from build123d import *

# Parameters (mm, degrees)
F0_W      = 36
F0_H      = 54
F1_DEPTH  = 15
F2_W      = 36
F2_H      = 7
F3_DEPTH  = 44
F4_R      = 15
F5_DEPTH  = 22
F7_D      = 20
F8_W      = 5
F8_H      = 7
F9_DEPTH  = 9999
F10_W     = 7
F10_H     = 7
F11_DEPTH = 11


with BuildPart() as f1:
    # F0 (on Top) → F1 (new body)
    with BuildSketch(Plane.XY):
        with Locations((-55.876545, -46.366083)):
            Rectangle(F0_W, F0_H)
    extrude(amount=F1_DEPTH)

    # F2 (on face) → F3 (join)
    with BuildSketch(Plane.XY.offset(15)):
        with Locations((-55.876545, -22.866083)):
            Rectangle(F2_W, F2_H)
        with Locations((-55.876545, -69.866083)):
            Rectangle(F2_W, F2_H)
    extrude(amount=F3_DEPTH)

    # F4 (on face) → F5 (join)
    with BuildSketch(Plane.XY.offset(15)):
        with Locations((-55.876545, -46.366083)):
            Circle(F4_R)
    extrude(amount=F5_DEPTH)

    # F7 (through all)
    with Locations(Plane.XY.offset(37)):
        with Locations((-55.876545, -46.366083)):
            Hole(F7_D / 2)

    # F8 (on Right) → F9 (cut)
    with BuildSketch(Plane.YZ):
        with Locations((-48.684213, 33.802636)):
            Rectangle(F8_W, F8_H)
        with Locations((-43.684213, 33.802636)):
            Rectangle(F8_W, F8_H)
    extrude(amount=-F9_DEPTH, mode=Mode.SUBTRACT)

    # F10 (on face) → F11 (join)
    with BuildSketch(Plane.XZ.offset(73.366083)):
        with Locations((-70.376545, 55.5)):
            Rectangle(F10_W, F10_H)
        with Locations((-41.376545, 55.5)):
            Rectangle(F10_W, F10_H)
    extrude(amount=F11_DEPTH)


solid = f1.part
Geometry: final body of the model. Coordinates: model frame, mm. A direction names the side the tool comes from. Give positions to 0.01 mm unless a question says otherwise; leave off trailing zeros. Loops run counter-clockwise (first coordinate to the right, second up) from the corner with the lowest first, then second, coordinate; pieces in that order, holes last. Notation, with made-up numbers: (0, 53.25) - (44, 53.25) arc R25 cw to (44, 85.25) - close; hole circle Ø2 at (41.5, -23.5). An arc over 180 degrees is marked (long way). Answer as CSV lines item,"result". Start each with the question number.
1. Reachability of faces 4 (the face through (-44.877, -79, 55)), 5 (the face through (-56, -26.366, 37)), 6 (the face through (-48.95, -59.67, 25.85)), 7 (the face through (-70, -79, 52)) from +Z, -Z, +X, -X, +Y, -Y: full face, straight path, thin tool, end or side. Return the list, or none.
2. Section C-C, the plane x = -59. Return loops of the section in (y, z), plus the area to 3 significant figures.
3. Ray query, L1, parallel to Y at x = -47, z = 53; L2, parallel to Y at x = -49, z = 17; L3, parallel to Z at x = -49.5, y = -36.5. Return the intervals inside material, ascending.
4. Section D-D, the plane z = 20. Return loops of the section in (x, y), plus the area to 3 significant figures.
5. Pin query (flat end, axial travel): P1, Ø18, axis at x = -57.5, z = 46, coming from the -Y side; P2, Ø5.5, axis at x = -42, y = -77, coming from the -Z side; P3, Ø1, axis at x = -50, y = -65.5, coming from the +Z side. Return the tip coordinate at first contact, or that it passes through.
6. Section A-A, the plane z = 43.5. Return loops of the section in (x, y).
7. Draft query along Y for faces 1 (the face through (-56, -73, 59)), 2 (the face through (-70, -84.366, 56)), 3 (the face through (-56, -36, 37)). Return one class per face: released by +Y, released by -Y, zero draft, split by the parting line, or undercut.
8. Section B-B, the plane y = -75. Return loops of the section in (x, z), plus the area to 3 significant figures.
Answers:
1,face 4,"+Z, -Z, -Y"
1,face 5,"+Z, +X, -X"
1,face 6,"+Z"
1,face 7,"-Z, +X, -X, -Y"
2,outline,"(-73.37, 0) - (-55.87, 0) - (-55.87, 37) - (-61.04, 37) - (-61.04, 15) - (-66.37, 15) - (-66.37, 59) - (-73.37, 59) - close; (-36.87, 0) - (-19.37, 0) - (-19.37, 59) - (-26.37, 59) - (-26.37, 15) - (-31.69, 15) - (-31.69, 37) - (-36.87, 37) - close"
2,area,"1,370 mm2"
3,L1,"y = -73.37 to -66.37, -26.37 to -19.37"
3,L2,"y = -73.37 to -66.37, -59.7 to -53.63, -39.11 to -33.04, -26.37 to -19.37"
3,L3,"z = 0 to 37"
4,outline,"(-73.88, -73.37) - (-37.88, -73.37) - (-37.88, -66.37) - (-73.88, -66.37) - close; (-73.88, -26.37) - (-37.88, -26.37) - (-37.88, -19.37) - (-73.88, -19.37) - close; circle Ø30 at (-55.88, -46.37); hole circle Ø20 at (-55.88, -46.37)"
4,area,"897 mm2"
5,P1,"stops at y = -73.37"
5,P2,"stops at z = 52"
5,P3,"stops at z = 15"
6,outline,"(-73.88, -73.37) - (-37.88, -73.37) - (-37.88, -66.37) - (-73.88, -66.37) - close; (-73.88, -26.37) - (-37.88, -26.37) - (-37.88, -19.37) - (-73.88, -19.37) - close"
7,face 1,"zero draft"
7,face 2,"released by -Y"
7,face 3,"undercut"
8,outline,"(-73.88, 52) - (-66.88, 52) - (-66.88, 59) - (-73.88, 59) - close; (-44.88, 52) - (-37.88, 52) - (-37.88, 59) - (-44.88, 59) - close"
8,area,"98.0 mm2"
